Work out the finished part from the listing and answer in its coordinate system (mm). Face numbers are marked on the shaded views. A direction names the side the tool comes from. Give positions to 0.01 mm unless a question says otherwise; leave off trailing zeros. Order: outer loops, then holes, each group sorted by start corner. A loop starts at its lowest first (then second) coordinate and runs counter-clockwise, first axis right, second up. Notation, with made-up numbers: M 31.5,13 L 83.5,13 A27 ccw 83.5,48 Z; hole C 40.5,-36.75 d9. An arc over 180 degrees is marked long. One line per item, written item: value.
from build123d import *

# Parameters (mm, degrees)
EXTRUDE_1_DEPTH     = 3
SKETCH_2_R          = 1
CUT_EXTRUDE_1_DEPTH = 3
EXTRUDE_2_DEPTH     = 3
CHAMFER_1_SIZE      = 0.25


with BuildPart() as part:
    # 草图1 → 凸台-拉伸1 (new body)
    with BuildSketch(Plane(origin=(0, 0, 0), x_dir=(1, 0, 0), z_dir=(0, 1, 0))):
        with BuildLine():
            Line((2, 1.5), (28, 1.5))
            ThreePointArc((28, 1.5), (32.5, 0), (28, -1.5))
            Line((28, -1.5), (2, -1.5))
            ThreePointArc((2, -1.5), (-2.5, 0), (2, 1.5))
        make_face()
    extrude(amount=EXTRUDE_1_DEPTH)

    # 草图2 → 切除-拉伸1 (cut)
    with BuildSketch(Plane(origin=(0, 0, 0), x_dir=(1, 0, 0), z_dir=(0, 1, 0))):
        with Locations(Location((0, 0, 0), (0, 0, 270))):
            Circle(SKETCH_2_R)
        with Locations(Location((30, 0, 0), (0, 0, 270))):
            Circle(SKETCH_2_R)
    extrude(amount=CUT_EXTRUDE_1_DEPTH, mode=Mode.SUBTRACT)

    # 草图3 → 凸台-拉伸2 (add)
    with BuildSketch(Plane(origin=(0, 0, 0), x_dir=(1, 0, 0), z_dir=(0, 1, 0))):
        with BuildLine():
            Line((4.5, 1.5), (0.578145188, 2.432231104))
            ThreePointArc((0.578145188, 2.432231104), (1.370755945, 2.090700395), (2, 1.5))
            Line((2, 1.5), (4.5, 1.5))
        make_face()
        with BuildLine():
            Line((4.5, -1.5), (0.578145188, -2.432231104))
            ThreePointArc((0.578145188, -2.432231104), (1.370755945, -2.090700395), (2, -1.5))
            Line((2, -1.5), (4.5, -1.5))
        make_face()
        with BuildLine():
            Line((28, 1.5), (25.5, 1.5))
            Line((25.5, 1.5), (29.421854812, 2.432231104))
            ThreePointArc((29.421854812, 2.432231104), (28.629244055, 2.090700395), (28, 1.5))
        make_face()
        with BuildLine():
            Line((25.5, -1.5), (29.421854812, -2.432231104))
            ThreePointArc((29.421854812, -2.432231104), (28.629244055, -2.090700395), (28, -1.5))
            Line((28, -1.5), (25.5, -1.5))
        make_face()
    extrude(amount=EXTRUDE_2_DEPTH)

    # 倒角1
    chamfer_1_edges = [part.edges().sort_by_distance(p)[0] for p in [
        (0, 0, -1),
        (0, 3, -1),
        (30, 0, -1),
        (30, 3, -1),
        (-2.5, 0, 0),
        (-2.5, 3, 0),
        (2.539072594, 0, -1.966115552),
        (2.539072594, 3, -1.966115552),
        (15, 0, 1.5),
        (15, 3, 1.5),
        (2.539072594, 0, 1.966115552),
        (2.539072594, 3, 1.966115552),
        (32.5, 0, 0),
        (32.5, 3, 0),
        (27.460927406, 0, 1.966115552),
        (27.460927406, 3, 1.966115552),
        (15, 0, -1.5),
        (15, 3, -1.5),
        (27.460927406, 0, -1.966115552),
        (27.460927406, 3, -1.966115552),
    ]]
    chamfer(chamfer_1_edges, length=CHAMFER_1_SIZE)


solid = part.part
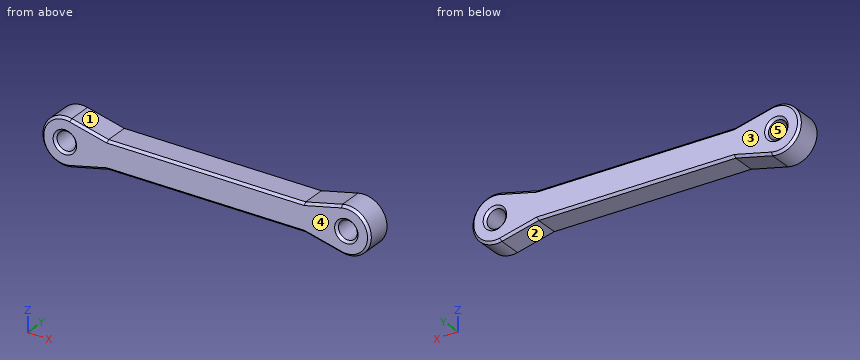
(1) Determine the mould class of the marked faces 4 and 5 for opening direction X: pulls with the +X half, pulls with the -X half, needs draft (parallel to the pull), parting line crosses it, or undercut.
Findings:
face 4: needs draft
face 5: undercut
(2) Which of the six approach directions +Z, -Z, +X, -X, +Y, -Y give full straight-line access (tool end or side, diameter ignored) to the marked faces 1, 2 and 3?
Findings:
face 1: +Z, +Y, -Y
face 2: -Z, +Y, -Y
face 3: +Z, -Z, +X, -X, +Y
(3) Given P1, Ø0.8, axis at x = 19.5, y = 2, coming from the -Z side; P2, Ø1.2, axis at x = 12.5, y = 1.5, coming from the +Z side, each flat-ended and moving along its own axis, determine where each tip first touches the part or whether it passes through.
Findings:
P1: stops at z = -1.5
P2: stops at z = 1.5
(4) Section C-C, the plane z = 0 is taken. Give the vertices of the cut face in (x, y).
Findings:
outline: M -2.5,0.25 L -2.25,0 L -1.25,0 L -1,0.25 L -1,2.75 L -1.25,3 L -2.25,3 L -2.5,2.75 Z; M 1,0.25 L 1.25,0 L 28.75,0 L 29,0.25 L 29,2.75 L 28.75,3 L 1.25,3 L 1,2.75 Z; M 31,0.25 L 31.25,0 L 32.25,0 L 32.5,0.25 L 32.5,2.75 L 32.25,3 L 31.25,3 L 31,2.75 Z
(5) Section D-D, the plane x = 25 is taken. Give the vertices of the cut face in (y, z), then the cut area to 4 significant figures.
Findings:
outline: M 0,-1.25 L 0.25,-1.5 L 2.75,-1.5 L 3,-1.25 L 3,1.25 L 2.75,1.5 L 0.25,1.5 L 0,1.25 Z
area: 8.875 mm^2
(6) Section B-B, the plane y = 0.95 is taken. Give the vertices of the cut face in (x, z).
Findings:
outline: M 0.58,-2.43 L 4.5,-1.5 L 25.5,-1.5 L 29.42,-2.43 A2.5 ccw long 29.42,2.43 L 25.5,1.5 L 4.5,1.5 L 0.58,2.43 A2.5 ccw long Z; hole C 0,0 d2; hole C 30,0 d2
(7) Section A-A, the plane x = 0 is taken. Give the vertices of the cut face in (y, z), then the cut area to 3 significant figures.
Findings:
outline: M 0,-2.25 L 0.25,-2.5 L 2.75,-2.5 L 3,-2.25 L 3,-1.25 L 2.75,-1 L 0.25,-1 L 0,-1.25 Z; M 0,1.25 L 0.25,1 L 2.75,1 L 3,1.25 L 3,2.25 L 2.75,2.5 L 0.25,2.5 L 0,2.25 Z
area: 8.75 mm^2
(8) Find the intervals of material crossed by probe 1 along X at (y, z) = (1.35, 0.1); probe 2 along X at (y, z) = (2.15, 0.45); probe 3 along Z at (x, y) = (12.5, 1.65), in increasing order. Write a range as from..to.
Findings:
probe 1: x = -2.5..-0.99, 0.99..29.01, 30.99..32.5
probe 2: x = -2.46..-0.89, 0.89..29.11, 30.89..32.46
probe 3: z = -1.5..1.5
